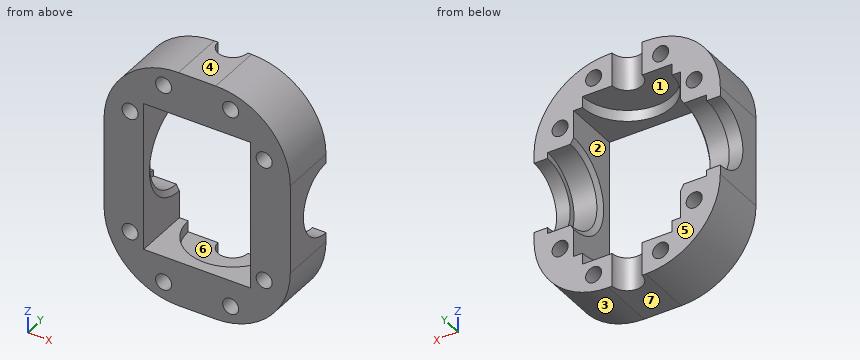
from build123d import *

# Parameters (mm, degrees)
SKETCH1_W             = 50
SKETCH1_H             = 64
SKETCH1_W_2           = 28.7
SKETCH1_H_2           = 40
BOSS_EXTRUDE1_DEPTH   = 15
SKETCH3_W             = 7
SKETCH3_H             = 11.1
SKETCH4_R             = 9.5
CUT_EXTRUDE2_DEPTH    = 51
SKETCH5_R             = 4
CUT_EXTRUDE3_DEPTH    = 65
SKETCH8_R             = 2.15
CUT_EXTRUDE6_DEPTH    = 16
FILLET1_R             = 20
CHAMFER1_SIZE         = 1.5
CHAMFER1_SIZE2        = 0.866025404
CHAMFER1_PART_2_SIZE  = 1.5
CHAMFER1_PART_2_SIZE2 = 0.866025404
SKETCH9_W             = 12
SKETCH9_H             = 3


with BuildPart() as part:
    # Sketch1 → Boss-Extrude1 (new body)
    with BuildSketch(Plane(origin=(0, 0, 0), x_dir=(1, 0, 0), z_dir=(0, 1, 0))):
        Rectangle(SKETCH1_W, SKETCH1_H)
        Rectangle(SKETCH1_W_2, SKETCH1_H_2, mode=Mode.SUBTRACT)
    extrude(amount=BOSS_EXTRUDE1_DEPTH)

    # Sketch3 → Cut-Revolve1 (revolve, cut)
    with BuildSketch(Plane(origin=(0, 15, 0), x_dir=(1, 0, 0), z_dir=(0, 1, 0))):
        with Locations((17.85, -5.55)):
            Rectangle(SKETCH3_W, SKETCH3_H)
        with Locations((-17.85, -5.55)):
            Rectangle(SKETCH3_W, SKETCH3_H)
    revolve(axis=Axis((14.35, 15, 0), (1, 0, 0)), mode=Mode.SUBTRACT)

    # Sketch4 → Cut-Extrude2 (cut, through all)
    with BuildSketch(Plane(origin=(25, 0, 0), x_dir=(0, 0, -1), z_dir=(1, 0, 0))):
        with Locations((0, 15)):
            Circle(SKETCH4_R)
    extrude(amount=-CUT_EXTRUDE2_DEPTH, mode=Mode.SUBTRACT)

    # Sketch5 → Cut-Extrude3 (cut, through all)
    with BuildSketch(Plane.XY.offset(32)):
        with Locations((0, 15)):
            Circle(SKETCH5_R)
    extrude(amount=-CUT_EXTRUDE3_DEPTH, mode=Mode.SUBTRACT)

    # Sketch8 → Cut-Extrude6 (cut, through all)
    with BuildSketch(Plane(origin=(0, 15, 0), x_dir=(1, 0, 0), z_dir=(0, 1, 0))):
        with Locations(Location((18, 16.5, 0), (0, 0, 270))):  # turned: the seam where the file's is
            Circle(SKETCH8_R)
        with Locations(Location((18, -16.5, 0), (0, 0, 270))):  # turned: the seam where the file's is
            Circle(SKETCH8_R)
        with Locations(Location((-18, -16.5, 0), (0, 0, 270))):  # turned: the seam where the file's is
            Circle(SKETCH8_R)
        with Locations(Location((-18, 16.5, 0), (0, 0, 270))):  # turned: the seam where the file's is
            Circle(SKETCH8_R)
        with Locations(Location((9, -27, 0), (0, 0, 270))):  # turned: the seam where the file's is
            Circle(SKETCH8_R)
        with Locations(Location((-9, -27, 0), (0, 0, 270))):  # turned: the seam where the file's is
            Circle(SKETCH8_R)
        with Locations(Location((-9, 27, 0), (0, 0, 270))):  # turned: the seam where the file's is
            Circle(SKETCH8_R)
        with Locations(Location((9, 27, 0), (0, 0, 270))):  # turned: the seam where the file's is
            Circle(SKETCH8_R)
    extrude(amount=-CUT_EXTRUDE6_DEPTH, mode=Mode.SUBTRACT)

    # Fillet1
    fillet1_edges = [part.edges().sort_by_distance(p)[0] for p in [
        (-25, 7.5, -32),
        (25, 7.5, -32),
        (25, 7.5, 32),
        (-25, 7.5, 32),
    ]]
    fillet(fillet1_edges, radius=FILLET1_R)

    # Chamfer1
    chamfer1_edges = [part.edges().sort_by_distance(p)[0] for p in [
        (14.35, 3.9, 0),
    ]]
    chamfer1_side = [part.faces().sort_by_distance(p)[0] for p in [
        (14.35, 0.427200187, 0),
    ]]
    chamfer(chamfer1_edges, length=CHAMFER1_SIZE, length2=CHAMFER1_SIZE2, reference=chamfer1_side[0])

    # Chamfer1 part 2
    chamfer1_part_2_edges = [part.edges().sort_by_distance(p)[0] for p in [
        (-14.35, 3.9, 0),
    ]]
    chamfer1_part_2_side = [part.faces().sort_by_distance(p)[0] for p in [
        (-14.35, 0.427200187, 0),
    ]]
    chamfer(chamfer1_part_2_edges, length=CHAMFER1_PART_2_SIZE, length2=CHAMFER1_PART_2_SIZE2, reference=chamfer1_part_2_side[0])

    # Sketch9 → Cut-Revolve2 (revolve, cut)
    with BuildSketch(Plane(origin=(0, 15, 0), x_dir=(1, 0, 0), z_dir=(0, 1, 0))):
        with Locations((-6, -21.5)):
            Rectangle(SKETCH9_W, SKETCH9_H)
        with Locations((-6, 21.5)):
            Rectangle(SKETCH9_W, SKETCH9_H)
    revolve(axis=Axis((0, 15, -29.871415895), (0, 0, 1)), mode=Mode.SUBTRACT)


solid = part.part
Model file for the job. Use its own axes, mm. Face numbers are marked on the shaded views. A direction names the side the tool comes from. Give positions to 0.01 mm unless a question says otherwise; leave off trailing zeros. Loops run counter-clockwise (first coordinate to the right, second up) from the corner with the lowest first, then second, coordinate; pieces in that order, holes last.
1) Wall check: line 1 (X direction, y = 8.25, z = -16.5); line 2 (Z direction, x = -0.5, y = 6.5); line 3 (X direction, y = 9.75, z = -27). Give the ranges that are in metal, low to high.
2) Pull direction Z, two halves, no side cores. Call the marked faces 4, 5, 6 and 7: +Z half, -Z half, draft (parallel to the pull), parting line (faces both ways), or undercut.
3) Saw through at B-B (z = 0). Write the cut outline in (x, y).
4) Saw through at D-D (z = 16.5). Write the cut outline in (x, y).
5) Saw through at C-C (x = -9). Write the cut outline in (y, z).
6) Flat gauge pins, fed straight in: pin 1 Ø3 at (x, y) = (8, 2.5) entering from -Z; pin 2 Ø6 at (x, y) = (-17, 8) entering from +Z; pin 3 Ø1 at (y, z) = (9, 23) entering from +X. Where does each tip first touch, or does it go through?
7) Tool access for the marked faces 1, 2 and 3: list every direction of +Z, -Z, +X, -X, +Y, -Y with a clear straight run to the whole face (end or side of a thin tool).
8) Saw through at A-A (x = 0). Write the cut outline in (y, z).
Answer block:
1. line 1: x = -24.49 to -20.15, -15.85 to -14.35, 14.35 to 15.85, 20.15 to 24.49
1. line 2: z = -32 to -23, 23 to 32
1. line 3: x = -18.23 to -11.15, -6.85 to 6.85, 11.15 to 18.23
2. face 4: +Z half
2. face 5: draft
2. face 6: undercut
2. face 7: -Z half
3. outline: (-25, 0) - (-14.35, 0) - (-14.35, 2.4) - (-15.22, 3.9) - (-21.35, 3.9) - (-21.35, 5.5) - (-25, 5.5) - close; (14.35, 0) - (25, 0) - (25, 5.5) - (21.35, 5.5) - (21.35, 3.9) - (15.22, 3.9) - (14.35, 2.4) - close
4. outline: (-24.49, 0) - (-20.15, 0) - (-20.15, 15) - (-24.49, 15) - close; (-15.85, 0) - (-14.35, 0) - (-14.35, 15) - (-15.85, 15) - close; (14.35, 0) - (15.85, 0) - (15.85, 15) - (14.35, 15) - close; (20.15, 0) - (24.49, 0) - (24.49, 15) - (20.15, 15) - close
5. outline: (0, -31.6) - (15, -31.6) - (15, -29.15) - (0, -29.15) - close; (0, -24.85) - (15, -24.85) - (15, -23) - (7.06, -23) - (7.06, -20) - (0, -20) - close; (0, 20) - (7.06, 20) - (7.06, 23) - (15, 23) - (15, 24.85) - (0, 24.85) - close; (0, 29.15) - (15, 29.15) - (15, 31.6) - (0, 31.6) - close
6. pin 1: stops at z = -31.94
6. pin 2: stops at z = 29.86
6. pin 3: stops at x = 22.02
7. face 1: +Y
7. face 2: +Y, -Y
7. face 3: -Z, +X, +Y, -Y
8. outline: (0, -32) - (11, -32) - (11, -23) - (3, -23) - (3, -20) - (0, -20) - close; (0, 20) - (3, 20) - (3, 23) - (11, 23) - (11, 32) - (0, 32) - close
